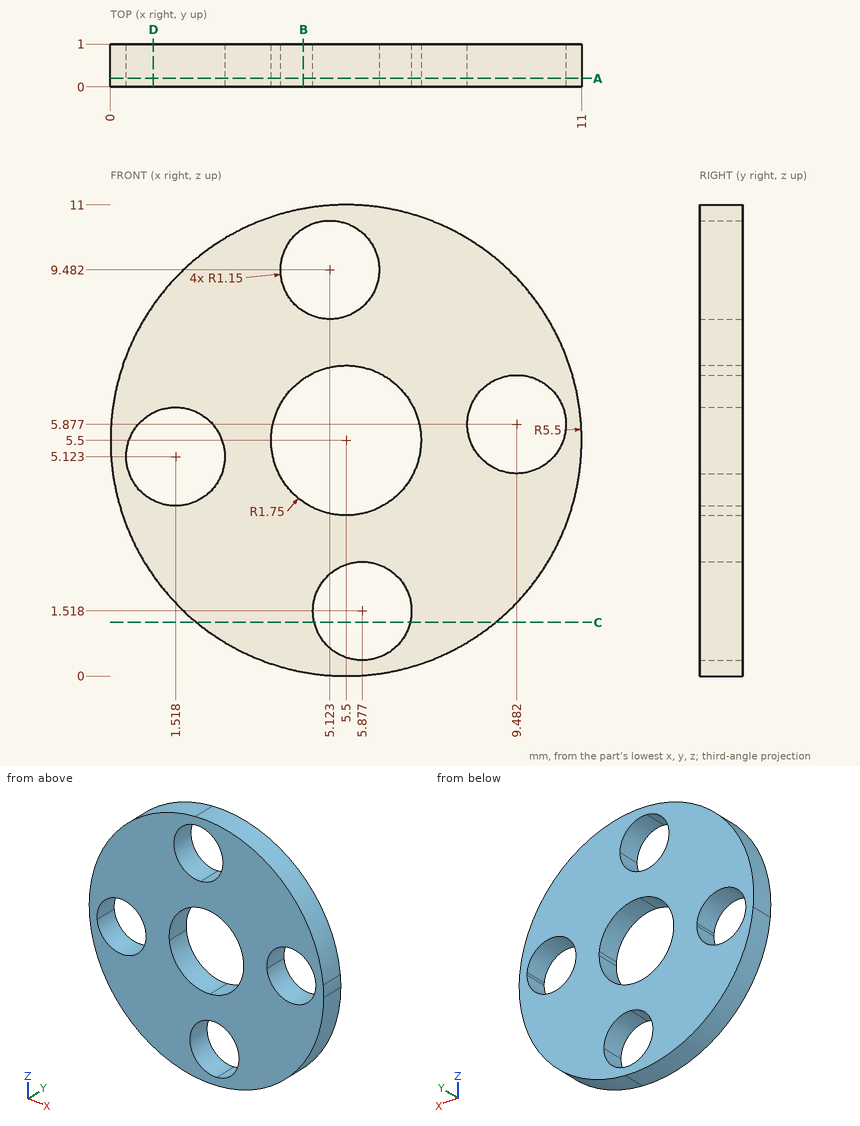
The drawing under review shows one solid part. Ordinate dimensions are in mm from its lowest x, y, z. Give positions to 0.01 mm unless a question says otherwise; leave off trailing zeros. Write each loop counter-clockwise with the first axis right and the second up, starting at its lowest first coordinate (ties: lowest second). Pieces come first, ordered by that corner, then holes. Notation, with made-up numbers: (39, -9.75) - (44, -9.75) arc R28 ccw to (44, 13.25) - close; hole circle Ø10 at (78, 13). An arc over 180 degrees is marked (long way). Answer in a Markdown table with one row per item. Add a question column.
1. We need section A-A on y = 0.2. State how many separate pieces and enclosed holes the cut face has, then the cut area to 3 significant figures.
2. We need section D-D on x = 1. Write out the cut boundary in (y, z).
3. We need section B-B on x = 4.5. Write out the cut boundary in (y, z).
4. Wall thickness on line 1 along Z through (x, y) = (4.5, 0.35) (1 decimal); line 2 along X through (y, z) = (0.5, 5) (1 decimal); line 3 along X through (y, z) = (0.3, 4.5) (1 decimal): over which ranges is each line inside the solid? List them lowest first. Write a range as [from, to].
5. We need section C-C on z = 1.25. Write out the cut boundary in (x, y).
Ans:
| question | item | result |
|---|---|---|
| 1 | separate pieces | 1 |
| 1 | enclosed holes | 5 |
| 1 | area | 68.8 mm^2 |
| 2 | outline | (0, 2.34) - (1, 2.34) - (1, 4.1) - (0, 4.1) - close; (0, 6.15) - (1, 6.15) - (1, 8.66) - (0, 8.66) - close |
| 3 | outline | (0, 0.09) - (1, 0.09) - (1, 4.06) - (0, 4.06) - close; (0, 6.94) - (1, 6.94) - (1, 8.52) - (0, 8.52) - close; (0, 10.45) - (1, 10.45) - (1, 10.91) - (0, 10.91) - close |
| 4 | line 1 | z = [0.1, 4.1], [6.9, 8.5], [10.4, 10.9] |
| 4 | line 2 | x = [0, 0.4], [2.7, 3.8], [7.2, 8.7], [10.2, 11] |
| 4 | line 3 | x = [0.1, 0.6], [2.5, 4.1], [6.9, 10.9] |
| 5 | outline | (2.01, 0) - (4.76, 0) - (4.76, 1) - (2.01, 1) - close; (7, 0) - (8.99, 0) - (8.99, 1) - (7, 1) - close |
